```python
from build123d import *

# Parameters (mm, degrees)
SKETCH1_R           = 25.4
BOSS_EXTRUDE1_DEPTH = 22.225
BOSS_EXTRUDE2_START = 22.225
SKETCH1_3_R         = 53.975
SKETCH1_3_R_2       = 0.5953125
BOSS_EXTRUDE2_DEPTH = 3.175
BOSS_EXTRUDE3_START = -19.05
SKETCH1_4_R         = 53.975
SKETCH1_4_R_2       = 25.4
SKETCH1_4_R_3       = 0.5953125
BOSS_EXTRUDE3_DEPTH = 3.175


with BuildPart() as part:
    # Sketch1 → Boss-Extrude1 (new, symmetric)
    with BuildSketch(Plane(origin=(0, 0, 0), x_dir=(0, 0, -1), z_dir=(1, 0, 0))):
        Circle(SKETCH1_R)
    extrude(amount=BOSS_EXTRUDE1_DEPTH, both=True)

    # Sketch1<3> → Boss-Extrude2 (add)
    with BuildSketch(Plane(origin=(0, 0, 0), x_dir=(0, 0, -1), z_dir=(1, 0, 0)).offset(BOSS_EXTRUDE2_START)):
        Circle(SKETCH1_3_R)
        with Locations((0, 50.8)):
            Circle(SKETCH1_3_R_2, mode=Mode.SUBTRACT)
        with Locations((7.571347122, 50.232605972)):
            Circle(SKETCH1_3_R_2, mode=Mode.SUBTRACT)
        with Locations((14.97356286, 48.543098534)):
            Circle(SKETCH1_3_R_2, mode=Mode.SUBTRACT)
        with Locations((22.041293947, 45.769218489)):
            Circle(SKETCH1_3_R_2, mode=Mode.SUBTRACT)
        with Locations((28.61665895, 41.972929735)):
            Circle(SKETCH1_3_R_2, mode=Mode.SUBTRACT)
        with Locations((34.552775079, 37.239035089)):
            Circle(SKETCH1_3_R_2, mode=Mode.SUBTRACT)
        with Locations((39.717039309, 31.673281934)):
            Circle(SKETCH1_3_R_2, mode=Mode.SUBTRACT)
        with Locations((43.994090512, 25.4)):
            Circle(SKETCH1_3_R_2, mode=Mode.SUBTRACT)
        with Locations((47.288386431, 18.559324038)):
            Circle(SKETCH1_3_R_2, mode=Mode.SUBTRACT)
        with Locations((49.526337939, 11.304063445)):
            Circle(SKETCH1_3_R_2, mode=Mode.SUBTRACT)
        with Locations((50.657952897, 3.796288754)):
            Circle(SKETCH1_3_R_2, mode=Mode.SUBTRACT)
        with Locations((50.657952897, -3.796288754)):
            Circle(SKETCH1_3_R_2, mode=Mode.SUBTRACT)
        with Locations((49.526337939, -11.304063445)):
            Circle(SKETCH1_3_R_2, mode=Mode.SUBTRACT)
        with Locations((47.288386431, -18.559324038)):
            Circle(SKETCH1_3_R_2, mode=Mode.SUBTRACT)
        with Locations((43.994090512, -25.4)):
            Circle(SKETCH1_3_R_2, mode=Mode.SUBTRACT)
        with Locations((39.717039309, -31.673281934)):
            Circle(SKETCH1_3_R_2, mode=Mode.SUBTRACT)
        with Locations((34.552775079, -37.239035089)):
            Circle(SKETCH1_3_R_2, mode=Mode.SUBTRACT)
        with Locations((28.61665895, -41.972929735)):
            Circle(SKETCH1_3_R_2, mode=Mode.SUBTRACT)
        with Locations((22.041293947, -45.769218489)):
            Circle(SKETCH1_3_R_2, mode=Mode.SUBTRACT)
        with Locations((14.97356286, -48.543098534)):
            Circle(SKETCH1_3_R_2, mode=Mode.SUBTRACT)
        with Locations((7.571347122, -50.232605972)):
            Circle(SKETCH1_3_R_2, mode=Mode.SUBTRACT)
        with Locations((0, -50.8)):
            Circle(SKETCH1_3_R_2, mode=Mode.SUBTRACT)
        with Locations((-7.571347122, -50.232605972)):
            Circle(SKETCH1_3_R_2, mode=Mode.SUBTRACT)
        with Locations((-14.97356286, -48.543098534)):
            Circle(SKETCH1_3_R_2, mode=Mode.SUBTRACT)
        with Locations((-22.041293947, -45.769218489)):
            Circle(SKETCH1_3_R_2, mode=Mode.SUBTRACT)
        with Locations((-28.61665895, -41.972929735)):
            Circle(SKETCH1_3_R_2, mode=Mode.SUBTRACT)
        with Locations((-34.552775079, -37.239035089)):
            Circle(SKETCH1_3_R_2, mode=Mode.SUBTRACT)
        with Locations((-39.717039309, -31.673281934)):
            Circle(SKETCH1_3_R_2, mode=Mode.SUBTRACT)
        with Locations((-43.994090512, -25.4)):
            Circle(SKETCH1_3_R_2, mode=Mode.SUBTRACT)
        with Locations((-47.288386431, -18.559324038)):
            Circle(SKETCH1_3_R_2, mode=Mode.SUBTRACT)
        with Locations((-49.526337939, -11.304063445)):
            Circle(SKETCH1_3_R_2, mode=Mode.SUBTRACT)
        with Locations((-50.657952897, -3.796288754)):
            Circle(SKETCH1_3_R_2, mode=Mode.SUBTRACT)
        with Locations((-50.657952897, 3.796288754)):
            Circle(SKETCH1_3_R_2, mode=Mode.SUBTRACT)
        with Locations((-49.526337939, 11.304063445)):
            Circle(SKETCH1_3_R_2, mode=Mode.SUBTRACT)
        with Locations((-47.288386431, 18.559324038)):
            Circle(SKETCH1_3_R_2, mode=Mode.SUBTRACT)
        with Locations((-43.994090512, 25.4)):
            Circle(SKETCH1_3_R_2, mode=Mode.SUBTRACT)
        with Locations((-39.717039309, 31.673281934)):
            Circle(SKETCH1_3_R_2, mode=Mode.SUBTRACT)
        with Locations((-34.552775079, 37.239035089)):
            Circle(SKETCH1_3_R_2, mode=Mode.SUBTRACT)
        with Locations((-28.61665895, 41.972929735)):
            Circle(SKETCH1_3_R_2, mode=Mode.SUBTRACT)
        with Locations((-22.041293947, 45.769218489)):
            Circle(SKETCH1_3_R_2, mode=Mode.SUBTRACT)
        with Locations((-14.97356286, 48.543098534)):
            Circle(SKETCH1_3_R_2, mode=Mode.SUBTRACT)
        with Locations((-7.571347122, 50.232605972)):
            Circle(SKETCH1_3_R_2, mode=Mode.SUBTRACT)
    extrude(amount=-BOSS_EXTRUDE2_DEPTH)

    # Sketch1<4> → Boss-Extrude3 (add)
    with BuildSketch(Plane(origin=(0, 0, 0), x_dir=(0, 0, -1), z_dir=(1, 0, 0)).offset(BOSS_EXTRUDE3_START)):
        Circle(SKETCH1_4_R)
        Circle(SKETCH1_4_R_2, mode=Mode.SUBTRACT)
        with Locations((0, 50.8)):
            Circle(SKETCH1_4_R_3, mode=Mode.SUBTRACT)
        with Locations((7.571347122, 50.232605972)):
            Circle(SKETCH1_4_R_3, mode=Mode.SUBTRACT)
        with Locations((14.97356286, 48.543098534)):
            Circle(SKETCH1_4_R_3, mode=Mode.SUBTRACT)
        with Locations((22.041293947, 45.769218489)):
            Circle(SKETCH1_4_R_3, mode=Mode.SUBTRACT)
        with Locations((28.61665895, 41.972929735)):
            Circle(SKETCH1_4_R_3, mode=Mode.SUBTRACT)
        with Locations((34.552775079, 37.239035089)):
            Circle(SKETCH1_4_R_3, mode=Mode.SUBTRACT)
        with Locations((39.717039309, 31.673281934)):
            Circle(SKETCH1_4_R_3, mode=Mode.SUBTRACT)
        with Locations((43.994090512, 25.4)):
            Circle(SKETCH1_4_R_3, mode=Mode.SUBTRACT)
        with Locations((47.288386431, 18.559324038)):
            Circle(SKETCH1_4_R_3, mode=Mode.SUBTRACT)
        with Locations((49.526337939, 11.304063445)):
            Circle(SKETCH1_4_R_3, mode=Mode.SUBTRACT)
        with Locations((50.657952897, 3.796288754)):
            Circle(SKETCH1_4_R_3, mode=Mode.SUBTRACT)
        with Locations((50.657952897, -3.796288754)):
            Circle(SKETCH1_4_R_3, mode=Mode.SUBTRACT)
        with Locations((49.526337939, -11.304063445)):
            Circle(SKETCH1_4_R_3, mode=Mode.SUBTRACT)
        with Locations((47.288386431, -18.559324038)):
            Circle(SKETCH1_4_R_3, mode=Mode.SUBTRACT)
        with Locations((43.994090512, -25.4)):
            Circle(SKETCH1_4_R_3, mode=Mode.SUBTRACT)
        with Locations((39.717039309, -31.673281934)):
            Circle(SKETCH1_4_R_3, mode=Mode.SUBTRACT)
        with Locations((34.552775079, -37.239035089)):
            Circle(SKETCH1_4_R_3, mode=Mode.SUBTRACT)
        with Locations((28.61665895, -41.972929735)):
            Circle(SKETCH1_4_R_3, mode=Mode.SUBTRACT)
        with Locations((22.041293947, -45.769218489)):
            Circle(SKETCH1_4_R_3, mode=Mode.SUBTRACT)
        with Locations((14.97356286, -48.543098534)):
            Circle(SKETCH1_4_R_3, mode=Mode.SUBTRACT)
        with Locations((7.571347122, -50.232605972)):
            Circle(SKETCH1_4_R_3, mode=Mode.SUBTRACT)
        with Locations((0, -50.8)):
            Circle(SKETCH1_4_R_3, mode=Mode.SUBTRACT)
        with Locations((-7.571347122, -50.232605972)):
            Circle(SKETCH1_4_R_3, mode=Mode.SUBTRACT)
        with Locations((-14.97356286, -48.543098534)):
            Circle(SKETCH1_4_R_3, mode=Mode.SUBTRACT)
        with Locations((-22.041293947, -45.769218489)):
            Circle(SKETCH1_4_R_3, mode=Mode.SUBTRACT)
        with Locations((-28.61665895, -41.972929735)):
            Circle(SKETCH1_4_R_3, mode=Mode.SUBTRACT)
        with Locations((-34.552775079, -37.239035089)):
            Circle(SKETCH1_4_R_3, mode=Mode.SUBTRACT)
        with Locations((-39.717039309, -31.673281934)):
            Circle(SKETCH1_4_R_3, mode=Mode.SUBTRACT)
        with Locations((-43.994090512, -25.4)):
            Circle(SKETCH1_4_R_3, mode=Mode.SUBTRACT)
        with Locations((-47.288386431, -18.559324038)):
            Circle(SKETCH1_4_R_3, mode=Mode.SUBTRACT)
        with Locations((-49.526337939, -11.304063445)):
            Circle(SKETCH1_4_R_3, mode=Mode.SUBTRACT)
        with Locations((-50.657952897, -3.796288754)):
            Circle(SKETCH1_4_R_3, mode=Mode.SUBTRACT)
        with Locations((-50.657952897, 3.796288754)):
            Circle(SKETCH1_4_R_3, mode=Mode.SUBTRACT)
        with Locations((-49.526337939, 11.304063445)):
            Circle(SKETCH1_4_R_3, mode=Mode.SUBTRACT)
        with Locations((-47.288386431, 18.559324038)):
            Circle(SKETCH1_4_R_3, mode=Mode.SUBTRACT)
        with Locations((-43.994090512, 25.4)):
            Circle(SKETCH1_4_R_3, mode=Mode.SUBTRACT)
        with Locations((-39.717039309, 31.673281934)):
            Circle(SKETCH1_4_R_3, mode=Mode.SUBTRACT)
        with Locations((-34.552775079, 37.239035089)):
            Circle(SKETCH1_4_R_3, mode=Mode.SUBTRACT)
        with Locations((-28.61665895, 41.972929735)):
            Circle(SKETCH1_4_R_3, mode=Mode.SUBTRACT)
        with Locations((-22.041293947, 45.769218489)):
            Circle(SKETCH1_4_R_3, mode=Mode.SUBTRACT)
        with Locations((-14.97356286, 48.543098534)):
            Circle(SKETCH1_4_R_3, mode=Mode.SUBTRACT)
        with Locations((-7.571347122, 50.232605972)):
            Circle(SKETCH1_4_R_3, mode=Mode.SUBTRACT)
    extrude(amount=-BOSS_EXTRUDE3_DEPTH)


solid = part.part
```
Geometry check sheet. Reference: the model listing, model coordinates, mm. A direction names the side the tool comes from. Round coordinates to 2 decimals unless told otherwise and drop trailing zeros. Loops run counter-clockwise (first coordinate to the right, second up) from the corner with the lowest first, then second, coordinate; pieces in that order, holes last. Notation, with made-up numbers: M 22,0 L 59,0 A20 cw 59,33 Z; hole C 60.25,79.25 d6. An arc over 180 degrees is marked long. Return JSON: item names as keys, results as strings. Group by question number.
(1) Section check B-B, the plane z = 11. Enter the section's corners in (x, y) (3 decimals).
(2) Set-up check for faces 1 (the face through (20.66, 36.48, 39.78)), 2 (the face through (-19.05, -11.2, -23.2)): record each of +Z, -Z, +X, -X, +Y, -Y from which the full face is reachable in a straight line by a thin tool's end or side.
(3) Section check C-C, the plane x = 2. Enter the section's corners in (y, z), and give its area (3 significant figures).
(4) Scan lines: line 1 along X through (y, z) = (29, -7.5) (3 decimals); line 2 along Z through (x, y) = (-3, -4.5). Record each from-to range of solid material in increasing order. Write a range as [from, to].
(5) Mould release check, pull along Z, two halves, no side actions. Record for faces 3 (the face through (-22.225, 1, 1)), 4 (the face through (-20.62, 36.48, 39.78)): pulls with the +Z half, pulls with the -Z half, needs draft (parallel to the pull), parting line crosses it, or undercut.
(6) Section check A-A, the plane y = 0. Enter the section's corners in (x, z) (3 decimals).
(7) Go/stop test with flat-tipped pins: pin 1 (1.1 mm diameter, centred on y = 3.8, z = -50.66, fed in from -X); pin 2 (10 mm diameter, centred on x = 16.5, z = -27.5, fed in from -Y) (3 decimals); pin 3 (1.5 mm diameter, centred on x = -14, z = 10, fed in from +Y); pin 4 (6 mm diameter, centred on x = 14.5, y = 23.5, fed in from -Z). Record where each tip stops, or that it passes through.
Data:
{
 "1": {"outline": "M -22.225,-52.842 L -19.05,-52.842 L -19.05,-22.895 L 19.05,-22.895 L 19.05,-52.842 L 22.225,-52.842 L 22.225,52.842 L 19.05,52.842 L 19.05,22.895 L -19.05,22.895 L -19.05,52.842 L -22.225,52.842 Z"},
 "2": {"face 1": "+X, -X", "face 2": "none"},
 "3": {"outline": "C 0,0 d50.8", "area": "2,030 mm²"},
 "4": {"line 1": "[-22.225, -19.05], [19.05, 22.225]", "line 2": "[-25, 25]"},
 "5": {"face 3": "needs draft", "face 4": "parting line crosses it"},
 "6": {"outline": "M -22.225,-53.975 L -19.05,-53.975 L -19.05,-25.4 L 19.05,-25.4 L 19.05,-53.975 L 22.225,-53.975 L 22.225,53.975 L 19.05,53.975 L 19.05,25.4 L -19.05,25.4 L -19.05,53.975 L -22.225,53.975 Z"},
 "7": {"pin 1": "through", "pin 2": "y = -48.735", "pin 3": "y = 23.66", "pin 4": "z = -15"}
}
